Here's how the part is built. I have some questions about the finished solid (model axes, mm). A direction names the side the tool comes from. Give positions to 0.01 mm unless a question says otherwise; leave off trailing zeros. Loops run counter-clockwise (first coordinate to the right, second up) from the corner with the lowest first, then second, coordinate; pieces in that order, holes last.
Q1. I need wall thicknesses on line 1 (Z direction, x = -5.1, y = 2.5); line 2 (Z direction, x = -5.75, y = 1.5); line 3 (X direction, y = -0.75, z = -6.75). Which ranges of each line are inside material? Lowest first, please.
Q2. Will these pins go through, and if not, where does the flat tip stop? P1, Ø0.8, axis at x = 3, y = -2.5, coming from the -Z side; P2, Ø1.5, axis at x = 1, z = -3, coming from the -Y side; P3, Ø0.8, axis at x = 8.5, y = -2, coming from the +Z side.
Q3. For faces 1 (the face through (0, 2.5, -0.5)), 2 (the face through (-5.38, 3.15, -5.01)), 3 (the face through (7, 2, -7)), which set-ups out of +Z, -Z, +X, -X, +Y, -Y let a thin tool reach every point of the face, with its end or its side?
Q4. If we section it at D-D (z = -5.5): Please give me the cut outline in (x, y), plus the area to 4 significant figures.
Q5. If we section it at A-A (y = -3): Please give me the cut outline in (x, z), plus the area to 3 significant figures.
Q6. If we section it at B-B (x = 8.25): Please give me the cut outline in (y, z).
Q7. If we section it at C-C (x = 3.75): Please give me the cut outline in (y, z), plus the area to 3 significant figures.
Q8. We'd pull the mould along Z, two halves only. Please class faces 4 (the face through (-3.458, 0.735, -3.444)), 5 (the face through (2, 5.2, -4)), 6 (the face through (4, 2, -8)): +Z half, -Z half, draft (parallel to the pull), parting line (faces both ways), or undercut.
from build123d import *

# Parameters (mm, degrees)
BOSS_EXTRU_1_DEPTH         = 5
BOSS_EXTRU_2_DEPTH         = 0.25
BOSS_EXTRU_3_DEPTH         = 2.94
ESQUISSE6_W                = 4.28
ESQUISSE6_H                = 4
ENL_V_MAT_EXTRU_1_DEPTH    = 0.7
ESQUISSE7_R                = 2.35
ESQUISSE7_R_2              = 1.85
BOSS_EXTRU_4_DEPTH         = 6
ESQUISSE8_R                = 1.2
BOSS_EXTRU_5_DEPTH         = 11
CONG_1_R                   = 1.1
ESQUISSE9_W                = 1.2
ESQUISSE9_H                = 4
BOSS_EXTRU_6_DEPTH         = 0.2
R_P_TITION_LIN_AIRE1_COUNT = 2
R_P_TITION_LIN_AIRE1_PITCH = 2.54
R_P_TITION_LIN_AIRE2_COUNT = 2
R_P_TITION_LIN_AIRE2_PITCH = 2.54


with BuildPart() as part:
    # Esquisse1 → Boss.-Extru.1 (new body)
    with BuildSketch(Plane(origin=(0, 0, 0), x_dir=(1, 0, 0), z_dir=(0, 1, 0))):
        Polygon((0, 0), (8, 0), (8, 1), (6.8, 1), (6.8, 7), (8, 7), (8, 8), (0, 8), align=None)
    extrude(amount=BOSS_EXTRU_1_DEPTH)

    # Esquisse4 → Boss.-Extru.2 (add, symmetric)
    with BuildSketch(Plane.XY.offset(-4)):
        Polygon((6.8, 4), (6.8, 1), (7.9, 1), (7.9, -4), (8.7, -4), (8.7, -0.6), (9.3, -0.6), (9.3, 4), align=None)
    boss_extru_2 = extrude(amount=BOSS_EXTRU_2_DEPTH, both=True)

    # Esquisse5 → Boss.-Extru.3 (add, symmetric)
    with BuildSketch(Plane.XY.offset(-4)):
        with BuildLine():
            Line((0, 5.2), (0, 0))
            Line((0, 0), (2.77, 0))
            ThreePointArc((2.77, 0), (3.264974747, -0.205025253), (3.47, -0.7))
            Line((3.47, -0.7), (3.47, -4))
            Line((3.47, -4), (2.97, -4))
            Line((2.97, -4), (2.97, -0.7))
            ThreePointArc((2.97, -0.7), (2.911421356, -0.558578644), (2.77, -0.5))
            Line((2.77, -0.5), (-0.2, -0.5))
            ThreePointArc((-0.2, -0.5), (-0.412132034, -0.412132034), (-0.5, -0.2))
            Line((-0.5, -0.2), (-0.5, 5.2))
            Line((-0.5, 5.2), (0, 5.2))
        make_face()
    extrude(amount=BOSS_EXTRU_3_DEPTH, both=True)

    # Esquisse6 → Enlèv. mat.-Extru.1 (cut)
    with BuildSketch(Plane(origin=(3.47, 0, 0), x_dir=(0, 0, -1), z_dir=(1, 0, 0))):
        with Locations((4, -2)):
            Rectangle(ESQUISSE6_W, ESQUISSE6_H)
    extrude(amount=-ENL_V_MAT_EXTRU_1_DEPTH, mode=Mode.SUBTRACT)

    # Esquisse7 → Boss.-Extru.4 (add)
    with BuildSketch(Plane.ZY.offset(0.5)):
        with Locations(Location((-4, 2.5, 0), (0, 0, 90))):
            Circle(ESQUISSE7_R)
        with Locations(Location((-4, 2.5, 0), (0, 0, 270))):
            Circle(ESQUISSE7_R_2, mode=Mode.SUBTRACT)
    extrude(amount=BOSS_EXTRU_4_DEPTH)

    # Esquisse8 → Boss.-Extru.5 (add)
    with BuildSketch(Plane.ZY.offset(0.5)):
        with Locations(Location((-4, 2.5, 0), (0, 0, 90))):
            Circle(ESQUISSE8_R)
    extrude(amount=BOSS_EXTRU_5_DEPTH)

    # Congé1
    cong_1_edges = [part.edges().sort_by_distance(p)[0] for p in [
        (-11.5, 1.3, -4),
    ]]
    fillet(cong_1_edges, radius=CONG_1_R)

    # Esquisse9 → Boss.-Extru.6 (add)
    with BuildSketch(Plane(origin=(0, 5, 0), x_dir=(1, 0, 0), z_dir=(0, 1, 0))):
        Polygon((0, 6.94), (5.2, 6.94), (6.3, 5.84), (6.3, 2.16), (5.2, 1.06), (0, 1.06), align=None)
        with Locations((4.7, 4)):
            Rectangle(ESQUISSE9_W, ESQUISSE9_H, mode=Mode.SUBTRACT)
    extrude(amount=BOSS_EXTRU_6_DEPTH)

    # Répétition linéaire1: Boss.-Extru.2 ×2
    with Locations(*[(0, 0, -i * R_P_TITION_LIN_AIRE1_PITCH) for i in range(1, R_P_TITION_LIN_AIRE1_COUNT)]):
        add(boss_extru_2)

    # Répétition linéaire2: Boss.-Extru.2 ×2
    with Locations(*[(0, 0, i * R_P_TITION_LIN_AIRE2_PITCH) for i in range(1, R_P_TITION_LIN_AIRE2_COUNT)]):
        add(boss_extru_2)


solid = part.part
Check sheet entries:
1. line 1: z = -6.35 to -5.85, -5.2 to -2.8, -2.15 to -1.65
1. line 2: z = -6.13 to -5.56, -4.66 to -3.34, -2.44 to -1.87
1. line 3: x = 2.97 to 3.47, 7.9 to 8.7
2. P1: stops at z = -6.94
2. P2: stops at y = -0.5
2. P3: stops at z = -1.21
3. face 1: +Z, -X, +Y, -Y
3. face 2: -X
3. face 3: +X, +Y, -Y
4. outline: (-6.5, 0.69) - (-0.5, 0.69) - (-0.5, -0.2) arc R0.3 ccw to (-0.2, -0.5) - (2.77, -0.5) - (2.77, 0) - (6.8, 0) - (6.8, 5) - (6.3, 5) - (6.3, 5.2) - (5.3, 5.2) - (5.3, 5) - (4.1, 5) - (4.1, 5.2) - (-0.5, 5.2) - (-0.5, 4.31) - (-6.5, 4.31) - (-6.5, 3.58) - (-0.5, 3.58) - (-0.5, 1.42) - (-6.5, 1.42) - close
4. area: 47.95 mm2
5. outline: (2.97, -6.94) - (3.47, -6.94) - (3.47, -6.14) - (2.97, -6.14) - close; (2.97, -1.86) - (3.47, -1.86) - (3.47, -1.06) - (2.97, -1.06) - close; (7.9, -6.79) - (8.7, -6.79) - (8.7, -6.29) - (7.9, -6.29) - close; (7.9, -4.25) - (8.7, -4.25) - (8.7, -3.75) - (7.9, -3.75) - close; (7.9, -1.71) - (8.7, -1.71) - (8.7, -1.21) - (7.9, -1.21) - close
5. area: 2.00 mm2
6. outline: (-4, -6.79) - (4, -6.79) - (4, -6.29) - (-4, -6.29) - close; (-4, -4.25) - (4, -4.25) - (4, -3.75) - (-4, -3.75) - close; (-4, -1.71) - (4, -1.71) - (4, -1.21) - (-4, -1.21) - close
7. outline: (0, -8) - (5, -8) - (5, -6.94) - (5.2, -6.94) - (5.2, -1.06) - (5, -1.06) - (5, 0) - (0, 0) - close
7. area: 41.2 mm2
8. face 4: undercut
8. face 5: draft
8. face 6: -Z half
